Geometry: final body of the model. Coordinates: model frame, mm. Face numbers are marked on the shaded views. A direction names the side the tool comes from. Coordinates: 2 decimals unless noted, no trailing zeros. Write each loop counter-clockwise with the first axis right and the second up, starting at its lowest first coordinate (ties: lowest second). Pieces come first, ordered by that corner, then holes. Notation, with made-up numbers: (11.25, 21.25) -> (15.25, 21.25) arc R20 cw to (15.25, 27.25) -> close; hole circle Ø8 at (29, 17.5). An arc over 180 degrees is marked (long way). One line per item, written item: value.
```python
from build123d import *

# Parameters (mm, degrees)
Y_KSEKLIK_EKSTR_ZYON1_DEPTH = 2.5
IZIM3_R                     = 2.116464506
KES_EKSTR_ZYON2_DEPTH       = 31
Y_KSEKLIK_EKSTR_ZYON3_DEPTH = 1.5


with BuildPart() as part:
    # Çizim1 → Yükseklik-Ekstrüzyon1 (new body, symmetric)
    with BuildSketch(Plane.XY):
        Polygon((20.082496858, 0), (18.413844112, 8.388883847), (13.661923129, 15.500636173), (6.550170803, 20.252557156), (-1.838713044, 21.921209901), (-10.22759689, 20.252557156), (-17.339349217, 15.500636173), (-22.0912702, 8.388883847), (-23.759922945, 0), (-22.0912702, -8.388883847), (-17.339349217, -15.500636173), (-10.22759689, -20.252557156), (-1.838713044, -21.921209901), (6.550170803, -20.252557156), (13.661923129, -15.500636173), (18.413844112, -8.388883847), align=None)
    extrude(amount=Y_KSEKLIK_EKSTR_ZYON1_DEPTH, both=True)

    # Çizim3 → Kes-Ekstrüzyon2 (cut)
    with BuildSketch(Plane(origin=(0, 0, -2.5), x_dir=(-1, 0, 0), z_dir=(0, 0, -1))):
        with Locations((1.838713044, 0)):
            Circle(IZIM3_R)
    extrude(amount=-KES_EKSTR_ZYON2_DEPTH, mode=Mode.SUBTRACT)

    # Çizim6 → Yükseklik-Ekstrüzyon3 (add, symmetric)
    with BuildSketch(Plane.XY):
        with BuildLine():
            ThreePointArc((-6.957303461, 25.732891749), (-4.672314924, 23.458692825), (-1.838713044, 21.921209901))
            Line((-1.838713044, 21.921209901), (-10.22759689, 20.252557156))
            ThreePointArc((-10.22759689, 20.252557156), (-8.198059352, 22.757378654), (-6.957303461, 25.732891749))
        make_face()
        with BuildLine():
            ThreePointArc((3.279877374, 25.732891749), (4.520633265, 22.757378654), (6.550170803, 20.252557156))
            Line((6.550170803, 20.252557156), (-1.838713044, 21.921209901))
            ThreePointArc((-1.838713044, 21.921209901), (0.994888837, 23.458692825), (3.279877374, 25.732891749))
        make_face()
        with BuildLine():
            ThreePointArc((12.737799217, 21.815292249), (12.745428626, 18.591459879), (13.661923129, 15.500636173))
            Line((13.661923129, 15.500636173), (6.550170803, 20.252557156))
            ThreePointArc((6.550170803, 20.252557156), (9.756446826, 20.588633667), (12.737799217, 21.815292249))
        make_face()
        with BuildLine():
            ThreePointArc((19.976579206, 14.576512261), (18.749920623, 11.59515987), (18.413844112, 8.388883847))
            Line((18.413844112, 8.388883847), (13.661923129, 15.500636173))
            ThreePointArc((13.661923129, 15.500636173), (16.752746836, 14.584141669), (19.976579206, 14.576512261))
        make_face()
        with BuildLine():
            ThreePointArc((23.894178705, 5.118590417), (21.619979781, 2.833601881), (20.082496858, 0))
            Line((20.082496858, 0), (18.413844112, 8.388883847))
            ThreePointArc((18.413844112, 8.388883847), (20.91866561, 6.359346308), (23.894178705, 5.118590417))
        make_face()
        with BuildLine():
            ThreePointArc((23.894178705, -5.118590417), (20.91866561, -6.359346308), (18.413844112, -8.388883847))
            Line((18.413844112, -8.388883847), (20.082496858, 0))
            ThreePointArc((20.082496858, 0), (21.619979781, -2.833601881), (23.894178705, -5.118590417))
        make_face()
        with BuildLine():
            ThreePointArc((19.976579206, -14.576512261), (16.752746836, -14.584141669), (13.661923129, -15.500636173))
            Line((13.661923129, -15.500636173), (18.413844112, -8.388883847))
            ThreePointArc((18.413844112, -8.388883847), (18.749920623, -11.59515987), (19.976579206, -14.576512261))
        make_face()
        with BuildLine():
            ThreePointArc((12.737799217, -21.815292249), (9.756446826, -20.588633667), (6.550170803, -20.252557156))
            Line((6.550170803, -20.252557156), (13.661923129, -15.500636173))
            ThreePointArc((13.661923129, -15.500636173), (12.745428626, -18.591459879), (12.737799217, -21.815292249))
        make_face()
        with BuildLine():
            ThreePointArc((3.279877374, -25.732891749), (0.994888837, -23.458692825), (-1.838713044, -21.921209901))
            Line((-1.838713044, -21.921209901), (6.550170803, -20.252557156))
            ThreePointArc((6.550170803, -20.252557156), (4.520633265, -22.757378654), (3.279877374, -25.732891749))
        make_face()
        with BuildLine():
            ThreePointArc((-6.957303461, -25.732891749), (-8.198059352, -22.757378654), (-10.22759689, -20.252557156))
            Line((-10.22759689, -20.252557156), (-1.838713044, -21.921209901))
            ThreePointArc((-1.838713044, -21.921209901), (-4.672314924, -23.458692825), (-6.957303461, -25.732891749))
        make_face()
        with BuildLine():
            ThreePointArc((-16.415225305, -21.815292249), (-16.422854713, -18.591459879), (-17.339349217, -15.500636173))
            Line((-17.339349217, -15.500636173), (-10.22759689, -20.252557156))
            ThreePointArc((-10.22759689, -20.252557156), (-13.433872913, -20.588633667), (-16.415225305, -21.815292249))
        make_face()
        with BuildLine():
            ThreePointArc((-23.654005293, -14.576512261), (-22.427346711, -11.59515987), (-22.0912702, -8.388883847))
            Line((-22.0912702, -8.388883847), (-17.339349217, -15.500636173))
            ThreePointArc((-17.339349217, -15.500636173), (-20.430172923, -14.584141669), (-23.654005293, -14.576512261))
        make_face()
        with BuildLine():
            ThreePointArc((-27.571604792, -5.118590417), (-25.297405869, -2.833601881), (-23.759922945, 0))
            Line((-23.759922945, 0), (-22.0912702, -8.388883847))
            ThreePointArc((-22.0912702, -8.388883847), (-24.596091698, -6.359346308), (-27.571604792, -5.118590417))
        make_face()
        with BuildLine():
            ThreePointArc((-27.571604793, 5.118590417), (-24.596091698, 6.359346308), (-22.0912702, 8.388883847))
            Line((-22.0912702, 8.388883847), (-23.759922945, 0))
            ThreePointArc((-23.759922945, 0), (-25.297405869, 2.833601881), (-27.571604793, 5.118590417))
        make_face()
        with BuildLine():
            ThreePointArc((-23.654005293, 14.576512261), (-20.430172923, 14.584141669), (-17.339349217, 15.500636173))
            Line((-17.339349217, 15.500636173), (-22.0912702, 8.388883847))
            ThreePointArc((-22.0912702, 8.388883847), (-22.427346711, 11.59515987), (-23.654005293, 14.576512261))
        make_face()
        with BuildLine():
            ThreePointArc((-16.415225305, 21.815292249), (-13.433872913, 20.588633667), (-10.22759689, 20.252557156))
            Line((-10.22759689, 20.252557156), (-17.339349217, 15.500636173))
            ThreePointArc((-17.339349217, 15.500636173), (-16.422854713, 18.591459879), (-16.415225305, 21.815292249))
        make_face()
    extrude(amount=Y_KSEKLIK_EKSTR_ZYON3_DEPTH, both=True)


solid = part.part
```
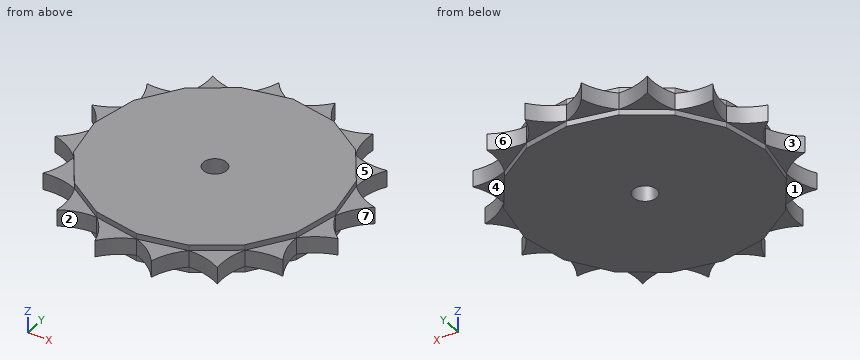
(1) Pull-direction query (X, two-part tool) for the marked faces 1, 2 and 3; classes: released by +X, released by -X, zero draft, split by the parting line, or undercut.
Responses:
face 1: zero draft
face 2: undercut
face 3: released by -X
(2) First-contact query: pin 1 (5 mm diameter, centred on x = -20.5, y = -12, fed in from +Z); pin 2 (1.6 mm diameter, centred on x = 22.5, y = -5.5, fed in from +Z); pin 3 (6 mm diameter, centred on x = -7, y = 24, fed in from -Z). Flat tips, straight axial feed; report the tip coordinate or a pass-through.
Responses:
pin 1: stops at z = 2.5
pin 2: stops at z = 1.5
pin 3: stops at z = -1.5
(3) Line query: line 1 (Y direction, x = -23.5, z = -0.6); line 2 (X direction, y = -21.5, z = -1.05); line 3 (Y direction, x = -10.5, z = 1.45). Output: solid intervals per line, ascending. Write a range as [from, to].
Responses:
line 1: y = [-14.56, -14.31], [-7.1, 7.1], [14.31, 14.56]
line 2: x = [-16.38, -15.84], [-9.07, 5.39], [12.17, 12.7]
line 3: y = [-20.25, 20.25]
(4) Reachability of the marked faces 4, 5, 6 and 7 from +Z, -Z, +X, -X, +Y, -Y: full face, straight path, thin tool, end or side. Return the list, or none.
Responses:
face 4: -Z, +X, +Y
face 5: +Z, +X, +Y
face 6: +Z, -Z, +Y
face 7: +Z, -Z, +X
(5) Section B-B (y = 1.5). Return the cut outline in (x, z), then the cut area to 3 significant figures.
Responses:
outline: (-24.44, -1.5) -> (-23.46, -1.5) -> (-23.46, -2.5) -> (-3.33, -2.5) -> (-3.33, 2.5) -> (-23.46, 2.5) -> (-23.46, 1.5) -> (-24.44, 1.5) -> close; (-0.35, -2.5) -> (19.78, -2.5) -> (19.78, -1.5) -> (20.77, -1.5) -> (20.77, 1.5) -> (19.78, 1.5) -> (19.78, 2.5) -> (-0.35, 2.5) -> close
area: 207 mm2
(6) Section D-D (x = -1). Return the cut outline in (y, z).
Responses:
outline: (-22.27, -1.5) -> (-21.75, -1.5) -> (-21.75, -2.5) -> (-1.94, -2.5) -> (-1.94, 2.5) -> (-21.75, 2.5) -> (-21.75, 1.5) -> (-22.27, 1.5) -> close; (1.94, -2.5) -> (21.75, -2.5) -> (21.75, -1.5) -> (22.27, -1.5) -> (22.27, 1.5) -> (21.75, 1.5) -> (21.75, 2.5) -> (1.94, 2.5) -> close
(7) Section C-C (x = 19). Return the cut outline in (y, z).
Responses:
outline: (-14.48, -1.5) -> (-12.44, -1.5) -> (-12.44, 1.5) -> (-14.48, 1.5) -> close; (-7.8, -1.5) -> (-5.44, -1.5) -> (-5.44, -2.5) -> (5.44, -2.5) -> (5.44, -1.5) -> (7.8, -1.5) -> (7.8, 1.5) -> (5.44, 1.5) -> (5.44, 2.5) -> (-5.44, 2.5) -> (-5.44, 1.5) -> (-7.8, 1.5) -> close; (12.44, -1.5) -> (14.48, -1.5) -> (14.48, 1.5) -> (12.44, 1.5) -> close
